Can you work these out from the model? Positions are in its coordinate system, mm. Face numbers are marked on the shaded views. A direction names the side the tool comes from. Round coordinates to 2 decimals unless told otherwise and drop trailing zeros. Order: outer loops, then holes, each group sorted by start corner. A loop starts at its lowest first (then second) coordinate and runs counter-clockwise, first axis right, second up. Notation, with made-up numbers: (-39, 54) -> (-5, 54) arc R17 ccw to (-5, 68) -> close; hole circle Ø9 at (9.25, -21). An arc over 180 degrees is marked (long way). One line per item, written item: value.
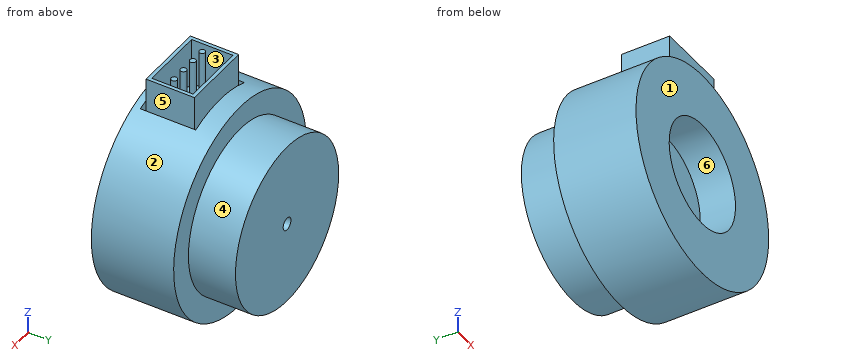
```python
from build123d import *

# Parameters (mm, degrees)
BOSS_EXTRU_1_DEPTH           = 2
BOSS_EXTRU_1_DEPTH_BACK      = 0.528751
ESQUISSE2_W                  = 6
ESQUISSE2_H                  = 4.109563502
ENL_V_MAT_EXTRU_1_DEPTH      = 2
ENL_V_MAT_EXTRU_1_DEPTH_BACK = 2
ESQUISSE3_W                  = 6.6
ESQUISSE3_H                  = 4.709563502
ESQUISSE3_W_2                = 6
ESQUISSE3_H_2                = 4.109563502


with BuildPart() as part:
    # Esquisse1 → R_volution1 (revolve)
    with BuildSketch(Plane.XY, mode=Mode.PRIVATE) as r_volution1_sk:
        Polygon((-4.5, 0), (-9, 0), (-9, 7), (-7, 7), (-7, 11), (-0.525, 11), (-0.525, 3), (-4.5, 3), align=None)
    revolve(r_volution1_sk.sketch.rotate(Axis((0, 0, 0), (0, 1, 0)), 270), axis=Axis((0, 0, 0), (0, 1, 0)))

    # Esquisse2 → Boss.-Extru.1 (add, two sides: drawn at the far end of the back side and taken through both)
    with BuildSketch(Plane.XY.offset(9).offset(-BOSS_EXTRU_1_DEPTH_BACK)):
        with Locations((0, 2.950126619)):
            Rectangle(ESQUISSE2_W, ESQUISSE2_H)
    extrude(amount=BOSS_EXTRU_1_DEPTH + BOSS_EXTRU_1_DEPTH_BACK)

    # Esquisse3 → Enl_v. mat.-Extru.1 (cut, two sides: drawn at the far end of the back side and taken through both)
    # profile 1 of 3: a face of its own
    with BuildSketch(Plane.XY.offset(9).offset(-ENL_V_MAT_EXTRU_1_DEPTH_BACK)):
        with Locations((0, 2.950126619)):
            Rectangle(ESQUISSE3_W, ESQUISSE3_H)
        with Locations((0, 2.950126619)):
            Rectangle(ESQUISSE3_W_2, ESQUISSE3_H_2, mode=Mode.SUBTRACT)
    # profile 2 of 3: a face of its own
    with BuildSketch(Plane.XY.offset(9).offset(-ENL_V_MAT_EXTRU_1_DEPTH_BACK)):
        with BuildLine():
            ThreePointArc((1.65, 2.595344868), (1.9, 2.845344868), (2.15, 2.595344868))
            Line((2.15, 2.595344868), (2.7, 2.595344868))
            Line((2.7, 2.595344868), (2.7, 4.70490837))
            Line((2.7, 4.70490837), (-2.7, 4.70490837))
            Line((-2.7, 4.70490837), (-2.7, 2.595344868))
            Line((-2.7, 2.595344868), (-2.160081964, 2.595344868))
            ThreePointArc((-2.160081964, 2.595344868), (-1.910081964, 2.845344868), (-1.660081964, 2.595344868))
            Line((-1.660081964, 2.595344868), (-0.890081964, 2.595344868))
            ThreePointArc((-0.890081964, 2.595344868), (-0.640081964, 2.845344868), (-0.390081964, 2.595344868))
            Line((-0.390081964, 2.595344868), (0.379918036, 2.595344868))
            ThreePointArc((0.379918036, 2.595344868), (0.629918036, 2.845344868), (0.879918036, 2.595344868))
            Line((0.879918036, 2.595344868), (1.65, 2.595344868))
        make_face()
    # profile 3 of 3: a face of its own
    with BuildSketch(Plane.XY.offset(9).offset(-ENL_V_MAT_EXTRU_1_DEPTH_BACK)):
        with BuildLine():
            Line((2.7, 2.595344868), (2.15, 2.595344868))
            ThreePointArc((2.15, 2.595344868), (1.9, 2.345344868), (1.65, 2.595344868))
            Line((1.65, 2.595344868), (0.879918036, 2.595344868))
            ThreePointArc((0.879918036, 2.595344868), (0.629918036, 2.345344868), (0.379918036, 2.595344868))
            Line((0.379918036, 2.595344868), (-0.390081964, 2.595344868))
            ThreePointArc((-0.390081964, 2.595344868), (-0.640081964, 2.345344868), (-0.890081964, 2.595344868))
            Line((-0.890081964, 2.595344868), (-1.660081964, 2.595344868))
            ThreePointArc((-1.660081964, 2.595344868), (-1.910081964, 2.345344868), (-2.160081964, 2.595344868))
            Line((-2.160081964, 2.595344868), (-2.7, 2.595344868))
            Line((-2.7, 2.595344868), (-2.7, 1.195344868))
            Line((-2.7, 1.195344868), (2.7, 1.195344868))
            Line((2.7, 1.195344868), (2.7, 2.595344868))
        make_face()
    extrude(amount=ENL_V_MAT_EXTRU_1_DEPTH + ENL_V_MAT_EXTRU_1_DEPTH_BACK, mode=Mode.SUBTRACT)


solid = part.part
```
Q1. I want a section at D-D on z = 7.25. List the corners of the cut face in (x, y) for me.
Answers below:
outline: (-5.33, 0) -> (5.33, 0) -> (5.33, 7) -> (-5.33, 7) -> close; (-3, 0.9) -> (3, 0.9) -> (3, 5) -> (-3, 5) -> close; circle Ø0.5 at (-1.91, 2.6); circle Ø0.5 at (-0.64, 2.6); circle Ø0.5 at (0.63, 2.6); circle Ø0.5 at (1.9, 2.6); hole (-3.3, 0.6) -> (3.3, 0.6) -> (3.3, 5.3) -> (-3.3, 5.3) -> close; hole (-2.7, 1.2) -> (2.7, 1.2) -> (2.7, 4.7) -> (-2.7, 4.7) -> close
Q2. We'd pull the mould along X, two halves only. Please class the marked faces 1, 2 and 3: released by +X, released by -X, zero draft, split by the parting line, or undercut.
Answers below:
face 1: zero draft
face 2: split by the parting line
face 3: undercut
Q3. I want a section at A-A on x = 0. List the corners of the cut face in (y, z) for me (3 decimals), plus the area to 3 significant figures.
Answers below:
outline: (0, -9) -> (7, -9) -> (7, -7) -> (11, -7) -> (11, -0.525) -> (3, -0.525) -> (3, -4.5) -> (0, -4.5) -> close; (0, 4.5) -> (3, 4.5) -> (3, 0.525) -> (11, 0.525) -> (11, 7) -> (7, 7) -> (7, 9) -> (5.305, 9) -> (5.305, 7) -> (5.005, 7) -> (5.005, 11) -> (4.705, 11) -> (4.705, 7) -> (1.195, 7) -> (1.195, 11) -> (0.895, 11) -> (0.895, 7) -> (0.595, 7) -> (0.595, 9) -> (0, 9) -> close
area: 140 mm^2
Q4. I want a section at B-B on z = 0. List the corners of the cut face in (x, y) for me (3 decimals).
Answers below:
outline: (-9, 0) -> (-4.5, 0) -> (-4.5, 3) -> (-0.525, 3) -> (-0.525, 11) -> (-7, 11) -> (-7, 7) -> (-9, 7) -> close; (0.525, 3) -> (4.5, 3) -> (4.5, 0) -> (9, 0) -> (9, 7) -> (7, 7) -> (7, 11) -> (0.525, 11) -> close
Q5. Will these pins go through, and if not, where does the flat tip stop? pin 1 Ø1.6 at (x, z) = (-0.5, 8.5) entering from +Y; pin 2 Ø1.8 at (y, z) = (3.5, 9) entering from -X; pin 3 Ø1.5 at (y, z) = (1.5, -2) entering from -X.
Answers below:
pin 1: y = 7
pin 2: x = -3.92
pin 3: x = -8.91
Q6. Please list where these lines run through material, in increasing order: line 1 along X through (y, z) = (2.25, 0); line 2 along X through (y, z) = (4.5, 0) (3 decimals); line 3 along Y through (x, z) = (0.75, 10.25).
Answers below:
line 1: -9 to -4.5, 4.5 to 9
line 2: -9 to -0.525, 0.525 to 9
line 3: 0.9 to 1.2, 2.38 to 2.81, 4.7 to 5
Q7. On a 3-axis mill with a long thin cutter (end or side, diameter ignored), from which of +Z, -Z, +X, -X, +Y, -Y can I reach the whole of each face in a straight line? I mean the marked faces 4, 5 and 6. Say none if no direction works.
Answers below:
face 4: +Y
face 5: +Z
face 6: -Y
Q8. I want a section at C-C on y = 2. List the corners of the cut face in (x, z) for me.
Answers below:
outline: (-3.3, 7) -> (-3.3, 8.37) arc R9 ccw (long way) to (3.3, 8.37) -> (3.3, 7) -> (3, 7) -> (3, 11) -> (2.7, 11) -> (2.7, 7) -> (-2.7, 7) -> (-2.7, 11) -> (-3, 11) -> (-3, 7) -> close; hole circle Ø9 at (0, 0)
